```python
from build123d import *

# Parameters (mm, degrees)
F1_DEPTH      = 25
F1_DEPTH_BACK = 25
F2_R          = 45.5
F3_DEPTH      = 23
F5_DEPTH      = 50.001
F6_R          = 2


with BuildPart() as f1:
    # F0 (on Right) → F1 (new body, two sides)
    with BuildSketch(Plane.YZ) as f1_sk:
        Polygon((3, 25), (0, 0), (25.179357, 0), (28.179357, 25), align=None)
    extrude(amount=F1_DEPTH)
    extrude(f1_sk.sketch, amount=-F1_DEPTH_BACK)

    # F2 (on face) → F3 (cut)
    with BuildSketch(Plane(origin=(0, 0, 0), x_dir=(1, 0, 0), z_dir=(0, -0.992877, 0.119145))):
        with Locations((0, 49.5)):
            Circle(F2_R)
    extrude(amount=-F3_DEPTH, mode=Mode.SUBTRACT)

    # F4 (on face) → F5 (cut, through all)
    with BuildSketch(Plane.YZ.offset(25)):
        Polygon((39.125659, 25), (24.232506, 26.787178), (22.087892, 8.915395), (36.981045, 7.128217), align=None)
    extrude(amount=-F5_DEPTH, mode=Mode.SUBTRACT)

    # F6
    f6_edges = [f1.edges().sort_by_distance(p)[0] for p in [
        (-25, 0.684105, 5.700878),
        (25, 0.684105, 5.700878),
        (25, 25.684744, 4.211563),
        (-25, 25.684744, 4.211563),
    ]]
    fillet(f6_edges, radius=F6_R)


solid = f1.part
```
Work out the finished part from the listing and answer in its coordinate system (mm). A direction names the side the tool comes from. Round coordinates to 2 decimals unless told otherwise and drop trailing zeros. Order: outer loops, then holes, each group sorted by start corner. A loop starts at its lowest first (then second) coordinate and runs counter-clockwise, first axis right, second up.
Q1. The mould has two halves that part along Y. Classify faces 1 (the flat face through (-25, 13, 4)), 2 (the cylindrical face through (24.43, 25.08, 4.22)), 3 (the cylindrical face through (24.4, 1.24, 5.55)), 4 (the cylindrical face through (-0.371, 11.735, 2.622)): pulls with the +Y half, pulls with the -Y half, needs draft (parallel to the pull), parting line crosses it, or undercut.
Solution:
face 1: needs draft
face 2: pulls with the +Y half
face 3: pulls with the -Y half
face 4: undercut
Q2. A cutting plane is placed at B-B, the plane x = -4. Determine the outline of the cut face in (y, z).
Solution:
outline: (0, 0) - (25.18, 0) - (26.19, 8.42) - (24.2, 8.66) - (23.33, 1.41) - (0.5, 4.15) - close
Q3. Find the intervals of material crossed by line 1 along X through (y, z) = (23.25, 6.5); line 2 along X through (y, z) = (20.5, 9); line 3 along X through (y, z) = (23.75, 4.25), in increasing order.
Solution:
line 1: x = -25 to -21.17, 21.17 to 25
line 2: x = -25 to -24.84, 24.84 to 25
line 3: x = -25 to 25
Q4. A tool of negligible diameter and unlimited length cuts with its end or side. For faces 5 (the flat face through (0.322, 25.678, 4.153)), 6 (the flat face through (-0.35, 23.864, 5.824)), from which of +Z, -Z, +X, -X, +Y, -Y can it reach the whole face along a straight path? Write none if from no direction.
Solution:
face 5: -Z, +X, -X, +Y
face 6: +Z
Q5. A cutting plane is placed at A-A, the plane x = 22.5. Determine the outline of the cut face in (y, z).
Solution:
outline: (0, 0) - (25.18, 0) - (26.19, 8.42) - (24.2, 8.66) - (24.02, 7.14) - (1.19, 9.88) - close
Q6. Given pin 1 Ø1.5 at (x, z) = (6.5, 4) entering from +Y; pin 2 Ø3 at (x, z) = (-16, 6) entering from -Y, each flat-ended and moving along its own axis, determine where each tip first touches the part or whether it passes through.
Solution:
pin 1: stops at y = 25.75
pin 2: stops at y = 0.54
